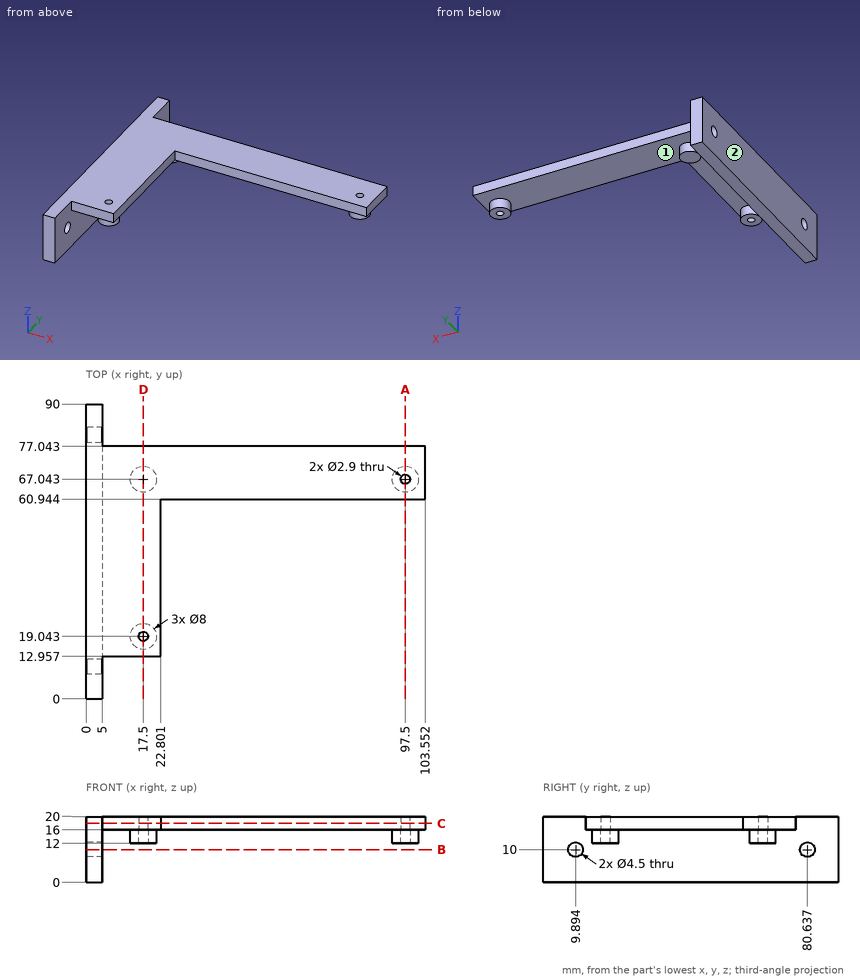
Geometry check sheet. Reference: drawing and pictorial views, mm from the part's lowest x, y, z. Give positions to 0.01 mm unless a question says otherwise; leave off trailing zeros. Write each loop counter-clockwise with the first axis right and the second up, starting at its lowest first coordinate (ties: lowest second). Pieces come first, ordered by that corner, then holes. Notation, with made-up numbers: (-37, 80.5) -> (-7, 80.5) arc R20 ccw to (-7, 111.5) -> close; hole circle Ø11 at (86, 58). An arc over 180 degrees is marked (long way). One line per item, written item: value. Start each with the question number.
Item 1: Section check D-D on x = 17.5. Record the cut outline in (y, z), then the cut area to 3 significant figures.
Item 2: Draft check along Y on the marked faces 1 and 2. Enter one of: +Y half, -Y half, draft (parallel to the pull), parting line (faces both ways), or undercut.
Item 3: Section check A-A on x = 97.5. Record the cut outline in (y, z).
Item 4: Material ranges on probe 1 along Y at (x, z) = (97.5, 17.4); probe 2 along Y at (x, z) = (17.5, 14.8); probe 3 along X at (y, z) = (70.5, 13.25) (1 decimal), recorded low to high. Write a range as from..to.
Item 5: Gauge pin test, flat ends, axial feed: pin 1 (12 mm diameter, centred on x = 29.5, z = 6.5, fed in from +Y); pin 2 (2 mm diameter, centred on x = 44, z = 18.5, fed in from -Y); pin 3 (10 mm diameter, centred on y = 70, z = 6, fed in from -X); pin 4 (1.5 mm diameter, centred on y = 16.5, z = 15.5, fed in from +X). Record the tip position at first contact, or that the pin passes through.
Item 6: Section check B-B on z = 10. Record the cut outline in (x, y), then the cut area to 3 significant figures.
Item 7: Section check C-C on z = 18. Record the cut outline in (x, y), then the cut area to 3 significant figures.
Results list:
1. outline: (12.96, 16) -> (15.04, 16) -> (15.04, 12) -> (17.59, 12) -> (17.59, 20) -> (12.96, 20) -> close; (20.49, 12) -> (23.04, 12) -> (23.04, 16) -> (63.04, 16) -> (63.04, 12) -> (71.04, 12) -> (71.04, 16) -> (77.04, 16) -> (77.04, 20) -> (20.49, 20) -> close
1. area: 297 mm²
2. face 1: undercut
2. face 2: draft
3. outline: (60.94, 16) -> (63.04, 16) -> (63.04, 12) -> (65.59, 12) -> (65.59, 20) -> (60.94, 20) -> close; (68.49, 12) -> (71.04, 12) -> (71.04, 16) -> (77.04, 16) -> (77.04, 20) -> (68.49, 20) -> close
4. probe 1: 60.94..65.59, 68.49..77.04
4. probe 2: 15.04..17.59, 20.49..23.04, 63.04..71.04
4. probe 3: 0..5, 15.5..19.5, 95.5..99.5
5. pin 1: through
5. pin 2: y = 60.94
5. pin 3: x = 0
5. pin 4: x = 22.8
6. outline: (0, 0) -> (5, 0) -> (5, 7.64) -> (0, 7.64) -> close; (0, 12.14) -> (5, 12.14) -> (5, 78.39) -> (0, 78.39) -> close; (0, 82.89) -> (5, 82.89) -> (5, 90) -> (0, 90) -> close
6. area: 405 mm²
7. outline: (0, 0) -> (5, 0) -> (5, 12.96) -> (22.8, 12.96) -> (22.8, 60.94) -> (103.55, 60.94) -> (103.55, 77.04) -> (5, 77.04) -> (5, 90) -> (0, 90) -> close; hole circle Ø2.9 at (17.5, 19.04); hole circle Ø2.9 at (97.5, 67.04)
7. area: 2,880 mm²
